Part print with two shaded views. Sizes in mm from the minimum x, y, z corner. A direction names the side the tool comes from. Coordinates: 2 decimals unless noted, no trailing zeros. Loops run counter-clockwise (first coordinate to the right, second up) from the corner with the lowest first, then second, coordinate; pieces in that order, holes last. Notation, with made-up numbers: (41, 7.25) -> (92, 7.25) arc R15 cw to (92, 25.25) -> close; hole circle Ø4 at (55, -1.75). An arc over 180 degrees is marked (long way). Answer as a JSON object with one key per item and string values. Group by question number.
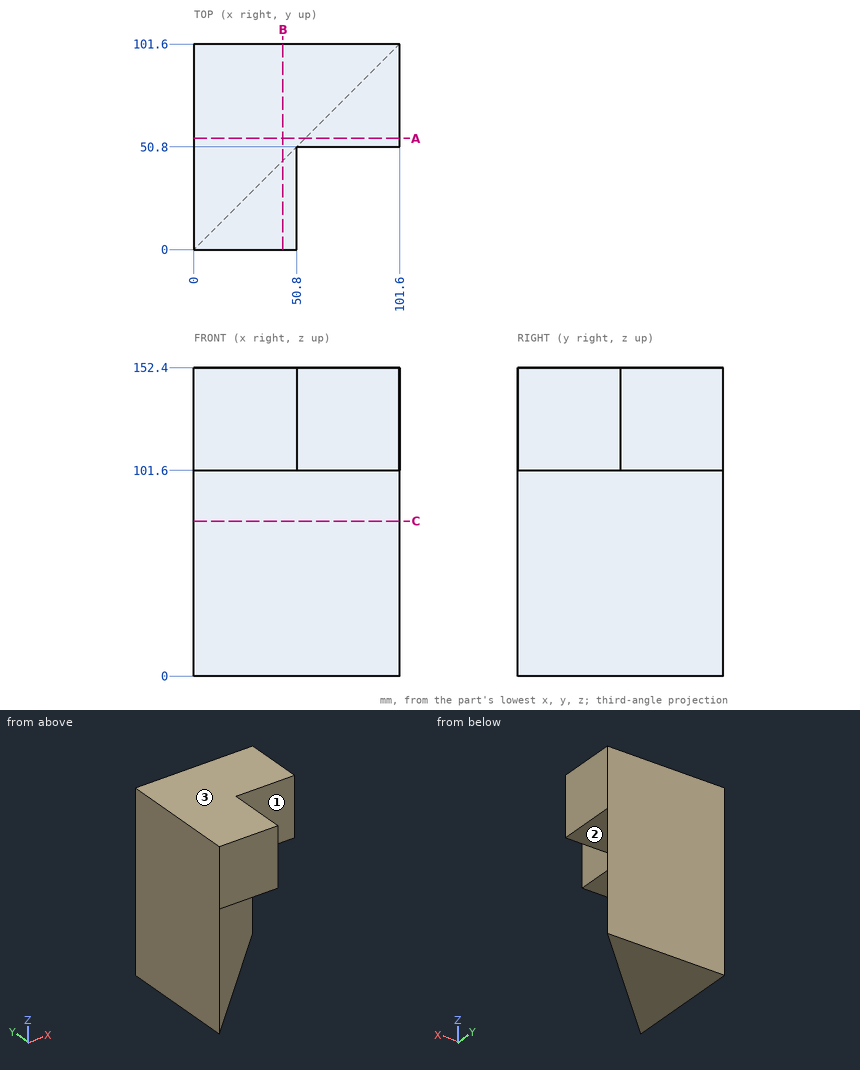
Item 1: 3-axis set-ups, long thin cutter, end or side, ignore diameter. For the marked faces 1, 2 and 3: which of +Z, -Z, +X, -X, +Y, -Y reach the whole face in a straight line?
Item 2: Band-saw the part on A-A, the plane y = 55. List the corners of the cut face in (x, z), and give its area (3 significant figures).
Item 3: Band-saw the part on C-C, the plane z = 76.5. List the corners of the cut face in (x, y), and give its area (3 significant figures).
Item 4: Flat gauge pins, fed straight in: P1, Ø1, axis at y = 18, z = 93, coming from the +X side; P2, Ø2, axis at x = 83.5, z = 106.5, coming from the -Y side; P3, Ø2, axis at x = 25.5, y = 17.5, coming from the -Z side. Where does each tip first touch, or does it go through?
Item 5: Band-saw the part on B-B, the plane x = 44. List the corners of the cut face in (y, z), and give its area (3 significant figures).
Item 6: Drill centre lines: L1, parallel to X at y = 6, z = 132; L2, parallel to Y at x = 87, z = 103; L3, parallel to X at y = 19.5, z = 70. Where is each one in solid material? Low to high.
Reply:
{
 "1": {"face 1": "+Z, -Z, +X, -Y", "face 2": "-Z, +X, -Y", "face 3": "+Z, +X, -X, +Y, -Y"},
 "2": {"outline": "(0, 0) -> (55, 0) -> (55, 101.6) -> (101.6, 101.6) -> (101.6, 152.4) -> (0, 152.4) -> close", "area": "10,700 mm²"},
 "3": {"outline": "(0, 0) -> (101.6, 101.6) -> (0, 101.6) -> close", "area": "5,160 mm²"},
 "4": {"P1": "x = 18.5", "P2": "y = 50.8", "P3": "z = 101.6"},
 "5": {"outline": "(0, 101.6) -> (44, 101.6) -> (44, 0) -> (101.6, 0) -> (101.6, 152.4) -> (0, 152.4) -> close", "area": "11,000 mm²"},
 "6": {"L1": "0 to 50.8", "L2": "50.8 to 101.6", "L3": "0 to 19.5"}
}
